Check sheet for the drawn part. Datum: minimum x, y, z corner. Units: mm. A direction names the side the tool comes from. Round coordinates to 2 decimals unless told otherwise and drop trailing zeros. Order: outer loops, then holes, each group sorted by start corner. A loop starts at its lowest first (then second) coordinate and runs counter-clockwise, first axis right, second up.
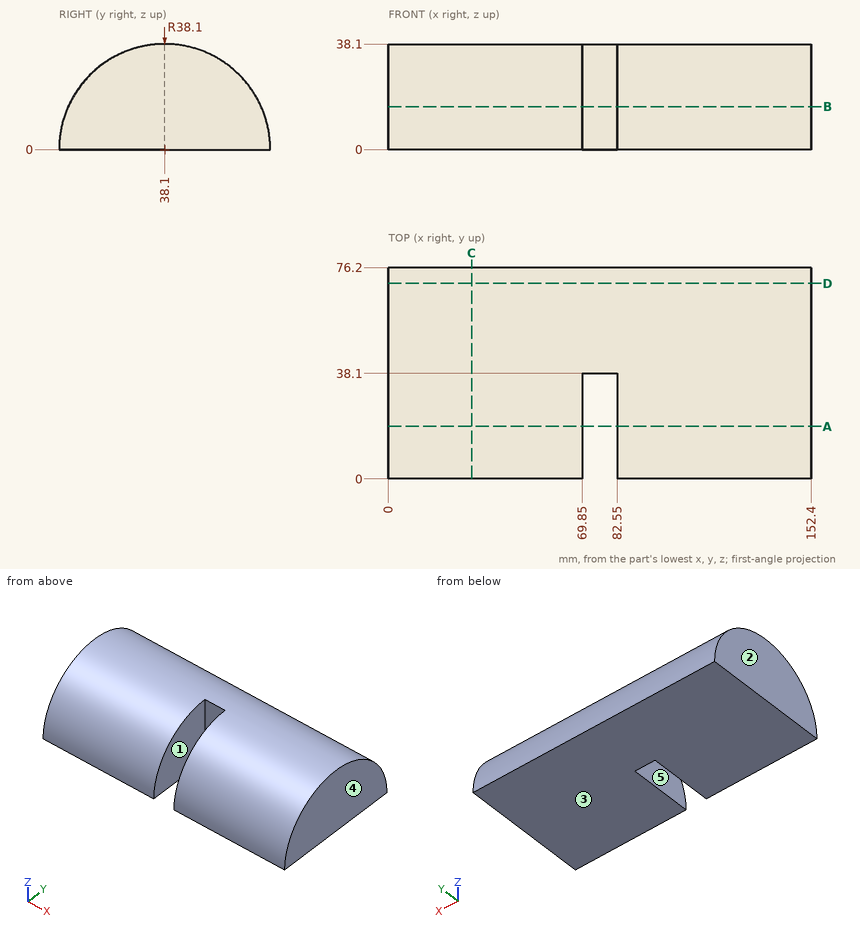
(1) Sectioned sample at C-C, the plane x = 30. Record the cut outline in (y, z), and give its area (3 significant figures).
Returned:
outline: (0, 0) - (76.2, 0) arc R38.1 ccw to start
area: 2,280 mm2
(2) Material ranges on line 1 (X direction, y = 14.5, z = 4); line 2 (Z direction, x = 135, y = 38); line 3 (Y direction, x = 76.5, z = 21), recorded low to high.
Returned:
line 1: x = 0 to 69.85, 82.55 to 152.4
line 2: z = 0 to 38.1
line 3: y = 38.1 to 69.89
(3) Draft check along X on the marked faces 3, 4 and 5. Enter one of: released by +X, released by -X, zero draft, split by the parting line, or undercut.
Returned:
face 3: zero draft
face 4: released by +X
face 5: undercut
(4) Sectioned sample at B-B, the plane z = 15.5. Record the cut outline in (x, y).
Returned:
outline: (0, 3.3) - (69.85, 3.3) - (69.85, 38.1) - (82.55, 38.1) - (82.55, 3.3) - (152.4, 3.3) - (152.4, 72.9) - (0, 72.9) - close
(5) Sectioned sample at A-A, the plane y = 19. Record the cut outline in (x, z), and give its area (3 significant figures).
Returned:
outline: (0, 0) - (69.85, 0) - (69.85, 32.97) - (0, 32.97) - close; (82.55, 0) - (152.4, 0) - (152.4, 32.97) - (82.55, 32.97) - close
area: 4,610 mm2
(6) Depth check by flat-ended pin: P1, Ø6, axis at x = 61, z = 6.5, coming from the -Y side; P2, Ø6.5, axis at x = 77, z = 26, coming from the -Y side. Enter the tip coordinate at first touch or a pass-through.
Returned:
P1: stops at y = 0.16
P2: stops at y = 38.1
(7) Set-up check for the marked faces 1 and 2: record each of +Z, -Z, +X, -X, +Y, -Y from which the full face is reachable in a straight line by a thin tool's end or side.
Returned:
face 1: +Z, -Z, -Y
face 2: +Z, -Z, -X, +Y, -Y
(8) Sectioned sample at D-D, the plane y = 70.5. Record the cut outline in (x, z), and give its area (3 significant figures).
Returned:
outline: (0, 0) - (152.4, 0) - (152.4, 20.05) - (0, 20.05) - close
area: 3,060 mm2
